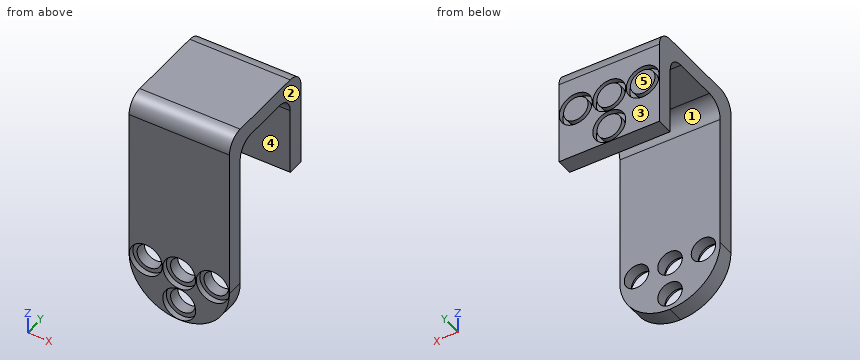
```python
from build123d import *

# Parameters (mm, degrees)
F1_DEPTH = 18
F2_R     = 2.95
F2_R_2   = 2.2
F3_DEPTH = 1
F4_R     = 3
F5_R     = 2.2
F6_DEPTH = 20.001
F5_R_2   = 2.95
F7_DEPTH = 1


with BuildPart() as f1:
    # F0 (on Right) → F1 (new body)
    with BuildSketch(Plane.YZ):
        with BuildLine():
            Line((10, 0), (10, 15))
            ThreePointArc((10, 15), (9.1213203436, 17.1213203436), (7, 18))
            Line((7, 18), (-7, 18))
            ThreePointArc((-7, 18), (-9.1213203436, 17.1213203436), (-10, 15))
            Line((-10, 15), (-10, -21))
            Line((-10, -21), (-7, -21))
            Line((-7, -21), (-7, 15))
            Line((-7, 15), (7, 15))
            Line((7, 15), (7, 0))
            Line((7, 0), (10, 0))
        make_face()
    extrude(amount=F1_DEPTH)

    # F2 (on face) → F3 (cut)
    with BuildSketch(Plane(origin=(0, 10, 0), x_dir=(-1, 0, 0), z_dir=(0, 1, 0))):
        with Locations((-14.9964041635, 8.9979103986)):
            Circle(F2_R)
        with Locations((-14.9964041635, 8.9979103986)):
            Circle(F2_R_2, mode=Mode.SUBTRACT)
        with Locations((-8.9964041635, 8.9979103986)):
            Circle(F2_R)
        with Locations((-8.9964041635, 8.9979103986)):
            Circle(F2_R_2, mode=Mode.SUBTRACT)
        with Locations((-2.9964041635, 8.9979103986)):
            Circle(F2_R)
        with Locations((-2.9964041635, 8.9979103986)):
            Circle(F2_R_2, mode=Mode.SUBTRACT)
        with Locations((-8.9964041635, 2.9979103986)):
            Circle(F2_R)
        with Locations((-8.9964041635, 2.9979103986)):
            Circle(F2_R_2, mode=Mode.SUBTRACT)
    extrude(amount=-F3_DEPTH, mode=Mode.SUBTRACT)

    # F4
    f4_edges = [f1.edges().sort_by_distance(p)[0] for p in [
        (9, 7, 15),
        (9, -7, 15),
    ]]
    fillet(f4_edges, radius=F4_R)

    # F5 (on face) → F6 (cut, through all)
    with BuildSketch(Plane.XZ.offset(10)):
        with BuildLine():
            ThreePointArc((18, -12), (15.3639610307, -18.3639610307), (9, -21))
            Line((9, -21), (18, -21))
            Line((18, -21), (18, -12))
        make_face()
        with BuildLine():
            ThreePointArc((9, -21), (2.6360389693, -18.3639610307), (0, -12))
            Line((0, -12), (0, -21))
            Line((0, -21), (9, -21))
        make_face()
        with Locations((3, -12)):
            Circle(F5_R)
        with Locations((9, -12)):
            Circle(F5_R)
        with Locations((15, -12)):
            Circle(F5_R)
        with Locations((9, -18)):
            Circle(F5_R)
    extrude(amount=-F6_DEPTH, mode=Mode.SUBTRACT)

    # F5 (on face) → F7 (cut)
    with BuildSketch(Plane.XZ.offset(10)):
        with Locations((3, -12)):
            Circle(F5_R_2)
        with Locations((3, -12)):
            Circle(F5_R, mode=Mode.SUBTRACT)
        with Locations((9, -12)):
            Circle(F5_R_2)
        with Locations((9, -12)):
            Circle(F5_R, mode=Mode.SUBTRACT)
        with Locations((15, -12)):
            Circle(F5_R_2)
        with Locations((15, -12)):
            Circle(F5_R, mode=Mode.SUBTRACT)
        with Locations((9, -18)):
            Circle(F5_R_2)
        with Locations((9, -18)):
            Circle(F5_R, mode=Mode.SUBTRACT)
    extrude(amount=-F7_DEPTH, mode=Mode.SUBTRACT)


solid = f1.part
```
Source: CAD feature listing. Evaluate the final solid. Frame: model axes, mm. Face numbers are marked on the shaded views. A direction names the side the tool comes from. Give positions to 0.01 mm unless a question says otherwise; leave off trailing zeros. Write each loop counter-clockwise with the first axis right and the second up, starting at its lowest first coordinate (ties: lowest second). Pieces come first, ordered by that corner, then holes.
1. First-contact query: pin 1 (1 mm diameter, centred on x = 11, y = 2, fed in from -Z); pin 2 (1 mm diameter, centred on y = -6, z = 12.5, fed in from +X); pin 3 (9 mm diameter, centred on x = 9.5, y = -0.5, fed in from -Z); pin 4 (4.5 mm diameter, centred on x = 15, z = -12, fed in from -Y). Flat tips, straight axial feed; report the tip coordinate or a pass-through.
2. Section query A-A (z = 2.5). Return the cut outline in (x, y), then the cut area to 3 significant figures.
3. Access query for the marked faces 4 and 5. Directions: +Z, -Z, +X, -X, +Y, -Y. A direction counts if a zero-diameter tool reaches every point of the face in a straight line with its end or side. Return the directions, or none.
4. Section query B-B (x = 16.5). Return the cut outline in (y, z), then the cut area to 3 significant figures.
5. Section query D-D (z = -18). Return the cut outline in (x, y), then the cut area to 3 significant figures.
6. Material intervals for line 1 along Y through (x, z) = (12.5, 8.5); line 2 along Z through (x, y) = (9, -7.4); line 3 along Y through (x, z) = (4.25, 9), sorted ascending.
7. Pull-direction query (Y, two-part tool) for the marked faces 1, 2 and 3; classes: +Y half, -Y half, draft (parallel to the pull), parting line (faces both ways), or undercut.
8. Section query C-C (y = 0.5). Return the cut outline in (x, z).
Output values:
1. pin 1: stops at z = 15
1. pin 2: passes through
1. pin 3: stops at z = 14.83
1. pin 4: stops at y = -9
2. outline: (0, -10) - (18, -10) - (18, -7) - (0, -7) - close; (0, 7) - (18, 7) - (18, 10) - (11.9, 10) - (11.9, 9) - (11.14, 9) - (11.14, 10) - (6.85, 10) - (6.85, 9) - (6.09, 9) - (6.09, 10) - (0, 10) - close
2. area: 106 mm2
3. face 4: -Z, +X, -X
3. face 5: +Z, -Z, +X, -X, +Y
4. outline: (-10, -16.97) - (-7, -16.97) - (-7, -13.61) - (-9, -13.61) - (-9, -14.54) - (-10, -14.54) - close; (-10, -9.46) - (-9, -9.46) - (-9, -10.39) - (-7, -10.39) - (-7, 12) arc R3 cw to (-4, 15) - (4, 15) arc R3 cw to (7, 12) - (7, 0) - (10, 0) - (10, 6.46) - (9, 6.46) - (9, 7.39) - (10, 7.39) - (10, 10.6) - (9, 10.6) - (9, 11.54) - (10, 11.54) - (10, 15) arc R3 ccw to (7, 18) - (-7, 18) arc R3 ccw to (-10, 15) - close
4. area: 188 mm2
5. outline: (2.29, -10) - (6.05, -10) - (6.05, -9) - (6.8, -9) - (6.8, -7) - (2.29, -7) - close; (11.2, -9) - (11.95, -9) - (11.95, -10) - (15.71, -10) - (15.71, -7) - (11.2, -7) - close
5. area: 25.5 mm2
6. line 1: y = -10 to -7, 7 to 9
6. line 2: z = -21 to -20.2, -15.8 to -14.2, -9.8 to 17.97
6. line 3: y = -10 to -7, 7 to 10
7. face 1: undercut
7. face 2: draft
7. face 3: +Y half
8. outline: (0, 15) - (18, 15) - (18, 18) - (0, 18) - close
